```python
from build123d import *

# Parameters (mm, degrees)
F0_W     = 23.5785879195
F0_H     = 17.130497843
F0_W_2   = 27.351161465
F0_H_2   = 5.9732412919
F1_DEPTH = 25.4


with BuildPart() as f1:
    # F0 (on Front) → F1 (new body)
    with BuildSketch(Plane.XZ):
        Polygon((-47.9431264102, 0), (-71.5217143297, 0), (-71.5217143297, -19.0233327448), (77.4949491024, -19.0233327448), (77.4949491024, 0), align=None)
        with Locations((-59.73242037, 8.5652489215)):
            Rectangle(F0_W, F0_H)
        Polygon((74.6655240655, 5.1840152591), (74.6655240655, 17.130497843), (43.5417890549, 17.130497843), (43.5417890549, 11.1572565511), (43.5417890549, 5.1840152591), align=None)
        with Locations((29.8662083223, 14.1438771971)):
            Rectangle(F0_W_2, F0_H_2)
        Polygon((-72.4648535252, 33.4783159196), (-72.4648535252, 17.130497843), (-71.5217143297, 17.130497843), (-47.9431264102, 17.130497843), (16.1906275898, 17.130497843), (43.5417890549, 17.130497843), (74.6655240655, 17.130497843), (74.6655240655, 33.4783159196), align=None)
    extrude(amount=F1_DEPTH)


solid = f1.part
```
The listing builds one solid part. Answer for the finished solid, in the listing's coordinates (mm). A direction names the side the tool comes from. Give positions to 0.01 mm unless a question says otherwise; leave off trailing zeros. Write each loop counter-clockwise with the first axis right and the second up, starting at its lowest first coordinate (ties: lowest second). Pieces come first, ordered by that corner, then holes. Notation, with made-up numbers: (14, -13.75) - (18, -13.75) arc R15 cw to (18, 14.25) - close; hole circle Ø4 at (62, 46.25). An arc over 180 degrees is marked (long way). Use one line per item in the form item = value. Start each with the question number.
1) Flat-ended cylindrical pins translate along their axes: pin 1 Ø5 at (y, z) = (-6.5, 20) entering from +X; pin 2 Ø7.5 at (y, z) = (-19, -2) entering from -X; pin 3 Ø0.8 at (x, y) = (-72, -11) entering from -Z. Find the tip coordinate at first contact, or state that the pin passes through.
2) Consider line 1 along Z through (x, y) = (9, -20); line 2 along Z through (x, y) = (17.5, -9); line 3 along X through (y, z) = (-15.25, -2.5). Determine where each line is inside the solid, lowest interval first. Write a range as from..to.
3) Find section B-B on z = 14. Determine the outline of the cut face in (x, y), plus the area to 3 significant figures.
4) Find section D-D on z = 22.5. Determine the outline of the cut face in (x, y), plus the area to 3 significant figures.
5) A tool of negligible diameter and unlimited length cuts with its end or side. For faces 1 (the face through (-71.522, -13, -1)), 2 (the face through (16, -13, 0)), 3 (the face through (2, -13, -19.023)), 4 (the face through (30, -13, 11.157)), 5 (the face through (74.666, -13, 19)), from which of +Z, -Z, +X, -X, +Y, -Y can it reach the whole face along a straight path? Write none if from no direction.
6) The mould has two halves that part along Z. Classify faces 6 (the face through (2, -13, 33.478)), 7 (the face through (77.495, -13, -10)), 8 (the face through (16.191, -13, 14)): pulls with the +Z half, pulls with the -Z half, needs draft (parallel to the pull), parting line crosses it, or undercut.
7) Find section A-A on x = 19.5. Determine the outline of the cut face in (y, z).
8) Find section C-C on y = -23.5. Determine the outline of the cut face in (x, z).
Geometry results:
q1.pin_1 = 74.67
q1.pin_2 = -71.52
q1.pin_3 = 17.13
q2.line_1 = -19.02..0, 17.13..33.48
q2.line_2 = -19.02..0, 11.16..33.48
q2.line_3 = -71.52..77.49
q3.outline = (-71.52, -25.4) - (-47.94, -25.4) - (-47.94, 0) - (-71.52, 0) - close; (16.19, -25.4) - (74.67, -25.4) - (74.67, 0) - (16.19, 0) - close
q3.area = 2,080 mm2
q4.outline = (-72.46, -25.4) - (74.67, -25.4) - (74.67, 0) - (-72.46, 0) - close
q4.area = 3,740 mm2
q5.face_1 = -Z, -X, +Y, -Y
q5.face_2 = +X, +Y, -Y
q5.face_3 = -Z, +X, -X, +Y, -Y
q5.face_4 = +Y, -Y
q5.face_5 = +Z, +X, +Y, -Y
q6.face_6 = pulls with the +Z half
q6.face_7 = needs draft
q6.face_8 = undercut
q7.outline = (-25.4, -19.02) - (0, -19.02) - (0, 0) - (-25.4, 0) - close; (-25.4, 11.16) - (0, 11.16) - (0, 33.48) - (-25.4, 33.48) - close
q8.outline = (-72.46, 17.13) - (-71.52, 17.13) - (-71.52, -19.02) - (77.49, -19.02) - (77.49, 0) - (-47.94, 0) - (-47.94, 17.13) - (16.19, 17.13) - (16.19, 11.16) - (43.54, 11.16) - (43.54, 5.18) - (74.67, 5.18) - (74.67, 33.48) - (-72.46, 33.48) - close
